```python
from build123d import *

# Parameters (mm, degrees)
F0_W     = 200
F0_H     = 200
F1_DEPTH = 150
F2_R     = 37.5
F3_DEPTH = 112
F4_R     = 47.5
F5_DEPTH = 8


with BuildPart() as f1:
    # F0 (on Top) → F1 (new body)
    with BuildSketch(Plane.XY):
        Rectangle(F0_W, F0_H)
    extrude(amount=F1_DEPTH)

    # F2 (on face) → F3 (cut)
    with BuildSketch(Plane.XY.offset(150)):
        Circle(F2_R)
    extrude(amount=-F3_DEPTH, mode=Mode.SUBTRACT)

    # F4 (on face) → F5 (cut)
    with BuildSketch(Plane.XY.offset(150)):
        Circle(F4_R)
    extrude(amount=-F5_DEPTH, mode=Mode.SUBTRACT)


solid = f1.part
```
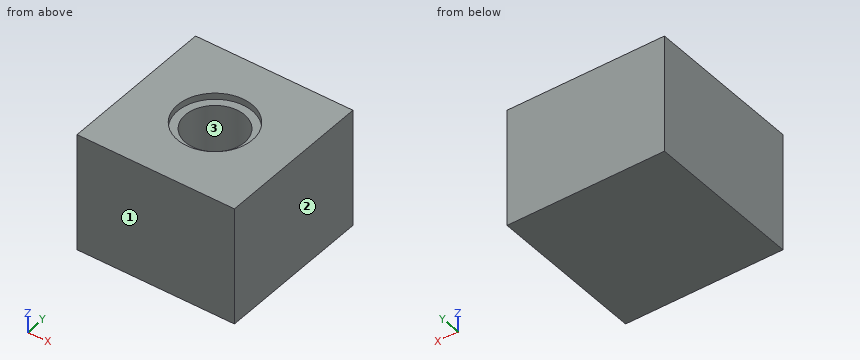
Check sheet for the modelled part. Datum: model origin and axes. Units: mm. Face numbers are marked on the shaded views. Give positions to 0.01 mm unless a question says otherwise; leave off trailing zeros. Order: outer loops, then holes, each group sorted by start corner. A loop starts at its lowest first (then second) coordinate and runs counter-clockwise, first axis right, second up. Notation, with made-up numbers: (54.5, 44) -> (101.5, 44) arc R28 cw to (101.5, 80) -> close; hole circle Ø3 at (20, 74.25). An arc over 180 degrees is marked (long way). Return JSON: item names as keys, results as strings.
1. Mould release check, pull along Y, two halves, no side actions. Record for the marked faces 1, 2 and 3: +Y half, -Y half, draft (parallel to the pull), parting line (faces both ways), or undercut.
From the geometry:
{"face 1": "-Y half", "face 2": "draft", "face 3": "undercut"}
2. Cross-section at A-A, the plane x = 0. Record the cut outline in (y, z), plus the area to 3 significant figures.
From the geometry:
{"outline": "(-100, 0) -> (100, 0) -> (100, 150) -> (47.5, 150) -> (47.5, 142) -> (37.5, 142) -> (37.5, 38) -> (-37.5, 38) -> (-37.5, 142) -> (-47.5, 142) -> (-47.5, 150) -> (-100, 150) -> close", "area": "21,400 mm^2"}
3. Cross-section at B-B, the plane z = 123. Record the cut outline in (x, y).
From the geometry:
{"outline": "(-100, -100) -> (100, -100) -> (100, 100) -> (-100, 100) -> close; hole circle Ø75 at (0, 0)"}
4. Material ranges on probe 1 along Y at (x, z) = (0, 73); probe 2 along Z at (x, y) = (24.5, -40); probe 3 along Y at (x, z) = (0, 145), recorded low to high. Write a range as [from, to].
From the geometry:
{"probe 1": "[-100, -37.5], [37.5, 100]", "probe 2": "[0, 142]", "probe 3": "[-100, -47.5], [47.5, 100]"}
